Geometry: final body of the model. Coordinates: model frame, mm. Coordinates: 2 decimals unless noted, no trailing zeros. Order: outer loops, then holes, each group sorted by start corner. A loop starts at its lowest first (then second) coordinate and runs counter-clockwise, first axis right, second up. Notation, with made-up numbers: M -31.75,-34 L 26.25,-34 A32 cw 26.25,-8 Z; hole C 86.5,-16 d8. An arc over 180 degrees is marked long. Use CSV: the item, a comma, the result in double quotes. Start each with the question number.
Q1. First-contact query: P1, Ø2.5, axis at x = 52, z = 33, coming from the -Y side; P2, Ø1.5, axis at y = 0.5, z = -2, coming from the -X side. Flat tips, straight axial feed; report the tip coordinate or a pass-through.
Q2. Section query B-B, the plane x = -18.5. Output: boundary loops of the cut face in (y, z).
Q3. Ray query, probe 1 along Z at (x, y) = (-27.5, 1.9); probe 2 along Z at (x, y) = (28, 1.65); probe 3 along X at (y, z) = (1.6, -8). Return the intervals inside material, ascending.
Q4. Section query D-D, the plane y = 0.5. State how many separate pieces and enclosed holes the cut face has, and give its area (3 significant figures).
Q5. Section query C-C, the plane z = -4.5. Output: boundary loops of the cut face in (x, y), and give its area (3 significant figures).
Q6. Section query A-A, the plane z = 33. Output: boundary loops of the cut face in (x, y).
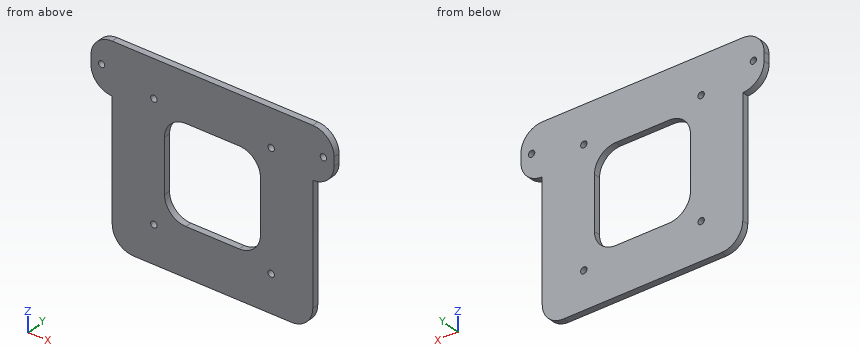
Autodesk Inventor part; units mm, degrees
ref_plane "YZ Plane" through (0, 0, 0) normal (1, 0, 0) x (0, 1, 0)
ref_plane "XZ Plane" through (0, 0, 0) normal (0, 1, 0) x (-1, 0, 0)
ref_plane "XY Plane" through (0, 0, 0) normal (0, 0, 1) x (1, 0, 0)
sketch "Sketch1" plane through (0, 0, 0) normal (0, 1, 0) x (-1, 0, 0)
  line L0 (-47, -45) -> (47, -45)
  line L1 (47, -45) -> (47, 45)
  line L2 (47, 45) -> (-47, 45)
  line L3 (-47, 45) -> (-47, -45)
  line L4 (-47, -45) -> (47, 45) construction
  line L5 (47, -45) -> (-47, 45) construction
  point P0 (0, 0)
  dimension "d0" = 94
  dimension "d1" = 90
extrude "Extrusion1" add sketch "Sketch1" along normal blind 3
sketch "Sketch2" plane through (0, 0, 0) normal (0, -1, 0) x (1, 0, 0)
  line L0 (-47, 45) -> (-57, 45)
  line L1 (-57, 45) -> (-57, 21)
  line L2 (-57, 21) -> (-47, 21)
  line L3 (-47, 21) -> (-47, 45)
  line L4 (47, -45) -> (-47, -45)
  point P0 (0, 0)
  dimension "d4" = 10
  dimension "d5" = 66
extrude "Extrusion2" add sketch "Sketch2" against normal blind 3
sketch "Sketch3" plane through (0, 0, 0) normal (0, -1, 0) x (1, 0, 0)
  line L0 (-30, 30) -> (30, 30) construction
  line L1 (30, 30) -> (30, -30) construction
  line L2 (30, -30) -> (-30, -30) construction
  line L3 (-30, -30) -> (-30, 30) construction
  line L4 (-30, 30) -> (30, -30) construction
  line L5 (30, 30) -> (-30, -30) construction
  circle A0 centre (-27.5, -27.5) radius 1.5
  circle A1 centre (27.5, -27.5) radius 1.5
  circle A2 centre (27.5, 27.5) radius 1.5
  circle A3 centre (-27.5, 27.5) radius 1.5
  point P0 (0, 0)
  dimension "d8" = 60
  dimension "d9" = 60
  dimension "d10" = 3
  dimension "d11" = 27.5
  dimension "d14" = 360
extrude "Extrusion3" cut sketch "Sketch3" against normal blind 3
sketch "Sketch4" plane through (0, 0, 0) normal (0, -1, 0) x (1, 0, 0)
  line L0 (22.5, 22.5) -> (-22.5, 22.5)
  line L1 (-22.5, 22.5) -> (-22.5, -22.5)
  line L2 (-22.5, -22.5) -> (22.5, -22.5)
  line L3 (22.5, -22.5) -> (22.5, 22.5)
  line L4 (22.5, 22.5) -> (-22.5, -22.5) construction
  line L5 (-22.5, 22.5) -> (22.5, -22.5) construction
  point P0 (0, 0)
  dimension "d18" = 45
  dimension "d19" = 45
extrude "Extrusion4" cut sketch "Sketch4" against normal blind 3
fillet "Fillet1" radius 10 3 edges at (-57, 1.5, 21) (-57, 1.5, 45) (-47, 1.5, -45)
mirror "Mirror1" about plane through (0, 0, 0) normal (1, 0, 0) of "Extrusion2", "Fillet1"
fillet "Fillet2" radius 10 4 edges at (-22.5, 1.5, -22.5) (22.5, 1.5, -22.5) (22.5, 1.5, 22.5) (-22.5, 1.5, 22.5)
sketch "Sketch5" plane through (0, 0, 0) normal (0, -1, 0) x (1, 0, 0)
  circle A0 centre (52, 33) radius 1.5
  line L0 (57, 35) -> (57, 31)
  point P0 (0, 0)
  point P1 (57, 33)
  dimension "d24" = 3
  dimension "d25" = 5
extrude "Extrusion5" cut sketch "Sketch5" against normal blind 3
mirror "Mirror2" about plane through (0, 0, 0) normal (1, 0, 0) of "Extrusion5"
properties part number "Bolt Cradel"
Responses:
1,P1,"passes through"
1,P2,"stops at x = -47"
2,outline,"M 0,-45 L 3,-45 L 3,-20.5 L 0,-20.5 Z; M 0,20.5 L 3,20.5 L 3,45 L 0,45 Z"
3,probe 1,"z = -45 to -29, -26 to 26, 29 to 45"
3,probe 2,"z = -45 to -28.91, -26.09 to 26.09, 28.91 to 45"
3,probe 3,"x = -47 to -22.5, 22.5 to 47"
4,separate pieces,"1"
4,enclosed holes,"7"
4,area,"6,830 mm²"
5,outline,"M -47,0 L -22.5,0 L -22.5,3 L -47,3 Z; M 22.5,0 L 47,0 L 47,3 L 22.5,3 Z"
5,area,"147 mm²"
6,outline,"M -57,0 L -53.5,0 L -53.5,3 L -57,3 Z; M -50.5,0 L 50.5,0 L 50.5,3 L -50.5,3 Z; M 53.5,0 L 57,0 L 57,3 L 53.5,3 Z"
